```python
from build123d import *

# Parameters (mm, degrees)
SKETCH_1_W          = 4
SKETCH_1_H          = 10
SKETCH_1_W_2        = 20
SKETCH_1_H_2        = 4
EXTRUDE_1_DEPTH     = 45
SKETCH_2_W          = 73
SKETCH_2_H          = 26
CUT_EXTRUDE_1_DEPTH = 5
FILLET_1_R          = 2
SKETCH_3_R          = 2.75
CUT_EXTRUDE_2_DEPTH = 5


with BuildPart() as part:
    # 스케치1 → 보스-돌출1 (new, symmetric)
    with BuildSketch(Plane.XY):
        Polygon((5.844814046, 44.543359129), (-6, 12), (-10, 12), (2.31272516, 45.828934348), align=None)
        with Locations((-8, 7)):
            Rectangle(SKETCH_1_W, SKETCH_1_H)
        Rectangle(SKETCH_1_W_2, SKETCH_1_H_2)
    extrude(amount=EXTRUDE_1_DEPTH, both=True)

    # 스케치2 → 컷-돌출1 (cut)
    with BuildSketch(Plane(origin=(-12.686947874, 4.61767139, 0), x_dir=(0, 0, 1), z_dir=(-0.9396926207859106, 0.34202014332566244, 0))):
        with Locations((0, 25.856110016)):
            Rectangle(SKETCH_2_W, SKETCH_2_H)
    extrude(amount=-CUT_EXTRUDE_1_DEPTH, mode=Mode.SUBTRACT)

    # 필렛1
    fillet_1_edges = [part.edges().sort_by_distance(p)[0] for p in [
        (4.078769603, 45.186146739, 45),
        (4.078769603, 45.186146739, -45),
        (-6, 12, 0),
        (-6, 2, 0),
        (-10, -2, 0),
        (-10, 12, 0),
        (2.368668886, 40.487683635, 36.5),
        (-6.52385484, 16.055675494, 36.5),
        (-6.52385484, 16.055675494, -36.5),
        (2.368668886, 40.487683635, -36.5),
    ]]
    fillet(fillet_1_edges, radius=FILLET_1_R)

    # 스케치3 → 컷-돌출2 (cut)
    with BuildSketch(Plane(origin=(0, 2, 0), x_dir=(1, 0, 0), z_dir=(0, 1, 0))):
        with Locations(Location((2, -30, 0), (0, 0, 270))):
            Circle(SKETCH_3_R)
        with Locations(Location((2, 15, 0), (0, 0, 270))):
            Circle(SKETCH_3_R)
    extrude(amount=-CUT_EXTRUDE_2_DEPTH, mode=Mode.SUBTRACT)


solid = part.part
```
Model file for the job. Use its own axes, mm. A direction names the side the tool comes from. Coordinates: 2 decimals unless noted, no trailing zeros. Write each loop counter-clockwise with the first axis right and the second up, starting at its lowest first coordinate (ties: lowest second). Pieces come first, ordered by that corner, then holes. Notation, with made-up numbers: (36, -34) - (56, -34) arc R26 ccw to (56, -6) - close; hole circle Ø8 at (57, 3). An arc over 180 degrees is marked (long way). Use a Markdown table: item, result. Add a question column.
Item 1: Band-saw the part on D-D, the plane z = 38. Write the cut outline in (x, y), and give its area (3 significant figures).
Item 2: Drop flat-ended pins along their axis: pin 1 (1.5 mm diameter, centred on x = 7.5, z = 35, fed in from +Y); pin 2 (2.5 mm diameter, centred on y = 6, z = -16.5, fed in from +X); pin 3 (6 mm diameter, centred on x = -1, y = 39.5, fed in from -Z); pin 4 (4.5 mm diameter, centred on x = 2, z = -15, fed in from -Y). Give the stop position or say it passes through.
Item 3: Two-plate mould, pull along Y, no slides. Class faces 1 (the face through (-6.549, 16.065, -0.483)), 2 (the face through (3, 2, 1)), 3 (the face through (2.121, 0.028, 27.253)), 4 (the face through (-9.4, -1.43, -0.63)): pulls with the +Y half, pulls with the -Y half, needs draft (parallel to the pull), parting line crosses it, or undercut.
Item 4: Band-saw the part on A-A, the plane z = -30.5. Write the cut outline in (x, y).
Item 5: Drill centre lines: line 1 along X through (y, z) = (0.4, 30); line 2 along Z through (x, y) = (0.75, 32); line 3 along Y through (x, z) = (8.5, 22.5). Where is each one in solid material? Low to high.
Item 6: Band-saw the part on C-C, the plane y = 31. Write the cut outline in (x, z).
Item 7: 3-axis set-ups, long thin cutter, end or side, ignore diameter. For faces 5 (the face through (-5.43, 2.6, -0.63)), 6 (the face through (-10, 6, 1)), 7 (the face through (-6.3, 16.58, -35.9)), 8 (the face through (2.34, 40.5, -0.48)), 9 (the face through (-4, 18, -45)): which of +Z, -Z, +X, -X, +Y, -Y reach the whole face in a straight line?
Item 8: Band-saw the part on B-B, the plane z = -15. Write the cut outline in (x, y).
A:
| question | item | result |
|---|---|---|
| 1 | outline | (-10, 0) arc R2 ccw to (-8, -2) - (10, -2) - (10, 2) - (-4, 2) arc R2 cw to (-6, 4) - (-6, 11.65) arc R2 cw to (-5.88, 12.33) - (5.84, 44.54) - (2.31, 45.83) - (-9.88, 12.33) arc R2 ccw to (-10, 11.65) - close |
| 1 | area | 253 mm² |
| 2 | pin 1 | stops at y = 2 |
| 2 | pin 2 | stops at x = -6 |
| 2 | pin 3 | stops at z = -45 |
| 2 | pin 4 | stops at y = 39.84 |
| 3 | face 1 | pulls with the +Y half |
| 3 | face 2 | undercut |
| 3 | face 3 | needs draft |
| 3 | face 4 | pulls with the -Y half |
| 4 | outline | (-10, 0) arc R2 ccw to (-8, -2) - (10, -2) - (10, 2) - (-4, 2) arc R2 cw to (-6, 4) - (-6, 11.65) arc R2 cw to (-5.88, 12.33) - (-4.76, 15.41) - (-8.29, 16.7) - (-9.88, 12.33) arc R2 ccw to (-10, 11.65) - close; (0.6, 41.13) - (4.13, 39.84) - (5.84, 44.54) - (2.31, 45.83) - close |
| 5 | line 1 | x = -10 to -0.75, 4.75 to 10 |
| 5 | line 2 | z = -45 to -36.5, 36.5 to 45 |
| 5 | line 3 | y = -2 to 2 |
| 6 | outline | (-3.08, -45) - (0.92, -45) - (0.92, -36.5) - (-3.08, -36.5) - close; (-3.08, 36.5) - (0.92, 36.5) - (0.92, 45) - (-3.08, 45) - close |
| 7 | face 5 | +Z, -Z, +X |
| 7 | face 6 | +Z, -Z, -X, +Y, -Y |
| 7 | face 7 | +X, +Y |
| 7 | face 8 | -X |
| 7 | face 9 | -Z, +X, -X, +Y, -Y |
| 8 | outline | (-10, 0) arc R2 ccw to (-8, -2) - (-0.75, -2) - (-0.75, 2) - (-4, 2) arc R2 cw to (-6, 4) - (-6, 11.65) arc R2 cw to (-5.88, 12.33) - (-4.76, 15.41) - (-8.29, 16.7) - (-9.88, 12.33) arc R2 ccw to (-10, 11.65) - close; (0.6, 41.13) - (4.13, 39.84) - (5.84, 44.54) - (2.31, 45.83) - close; (4.75, -2) - (10, -2) - (10, 2) - (4.75, 2) - close |
